Here's how the part is built. I have some questions about the finished solid (model axes, mm). A direction names the side the tool comes from. Round coordinates to 2 decimals unless told otherwise and drop trailing zeros. Order: outer loops, then holes, each group sorted by start corner. A loop starts at its lowest first (then second) coordinate and runs counter-clockwise, first axis right, second up. Notation, with made-up numbers: (72.25, 31) -> (121.25, 31) arc R24 ccw to (121.25, 57) -> close; hole circle Ø8 at (-38, 58). An arc over 180 degrees is marked (long way). Answer in a Markdown table with one row per item.
```python
from build123d import *

# Parameters (mm, degrees)
SKETCH2_W           = 16
SKETCH2_H           = 16
BOSS_EXTRUDE1_DEPTH = 1.7
SKETCH3_R           = 0.75
CUT_EXTRUDE1_DEPTH  = 1.7
SKETCH4_W           = 3
SKETCH4_H           = 3
BOSS_EXTRUDE2_DEPTH = 1
SKETCH5_W           = 0.710598353
SKETCH5_H           = 2.069095202
SKETCH5_H_2         = 1.860095687
BOSS_EXTRUDE3_DEPTH = 0.5
SKETCH6_R           = 1.65
CUT_EXTRUDE2_DEPTH  = 12.440716761


with BuildPart() as part:
    # Sketch2 → Boss-Extrude1 (new body)
    with BuildSketch(Plane(origin=(0, 0, 0), x_dir=(1, 0, 0), z_dir=(0, 1, 0))):
        Rectangle(SKETCH2_W, SKETCH2_H)
    extrude(amount=BOSS_EXTRUDE1_DEPTH)

    # Sketch3 → Cut-Extrude1 (cut)
    with BuildSketch(Plane(origin=(0, 1.7, 0), x_dir=(1, 0, 0), z_dir=(0, 1, 0))):
        with Locations(Location((-6.5, 6.35, 0), (0, 0, 270))):
            Circle(SKETCH3_R)
        with Locations(Location((-6.5, 3.81, 0), (0, 0, 270))):
            Circle(SKETCH3_R)
        with Locations(Location((-6.5, 1.27, 0), (0, 0, 270))):
            Circle(SKETCH3_R)
        with Locations(Location((-6.5, -1.27, 0), (0, 0, 270))):
            Circle(SKETCH3_R)
        with Locations(Location((-6.5, -3.81, 0), (0, 0, 270))):
            Circle(SKETCH3_R)
        with Locations(Location((-6.5, -6.35, 0), (0, 0, 270))):
            Circle(SKETCH3_R)
    extrude(amount=-CUT_EXTRUDE1_DEPTH, mode=Mode.SUBTRACT)

    # Sketch4 → Boss-Extrude2 (add)
    with BuildSketch(Plane(origin=(0, 1.7, 0), x_dir=(1, 0, 0), z_dir=(0, 1, 0))):
        Rectangle(SKETCH4_W, SKETCH4_H)
    extrude(amount=BOSS_EXTRUDE2_DEPTH)

    # Sketch5 → Boss-Extrude3 (add)
    with BuildSketch(Plane(origin=(0, 1.7, 0), x_dir=(1, 0, 0), z_dir=(0, 1, 0))):
        with Locations((0.571550994, 4.723389047)):
            Rectangle(SKETCH5_W, SKETCH5_H)
        with Locations((-0.428449007, 4.723389047)):
            Rectangle(SKETCH5_W, SKETCH5_H)
        with Locations((-1.01364765, -4.388989823)):
            Rectangle(SKETCH5_W, SKETCH5_H_2)
        with Locations((-0.013647649, -4.388989823)):
            Rectangle(SKETCH5_W, SKETCH5_H_2)
        with Locations((0.986352351, -4.388989823)):
            Rectangle(SKETCH5_W, SKETCH5_H_2)
    extrude(amount=BOSS_EXTRUDE3_DEPTH)

    # Sketch6 → Cut-Extrude2 (cut, through all)
    with BuildSketch(Plane(origin=(0, 1.7, 0), x_dir=(1, 0, 0), z_dir=(0, 1, 0))):
        with Locations(Location((5, 5.1, 0), (0, 0, 270))):
            Circle(SKETCH6_R)
        with Locations(Location((5, -5.1, 0), (0, 0, 90))):
            Circle(SKETCH6_R)
    extrude(amount=-CUT_EXTRUDE2_DEPTH, mode=Mode.SUBTRACT)


solid = part.part
```
1. Suppose I cut it at D-D on y = 1.2. State how many separate pieces and enclosed holes the cut face has, then the cut area to 3 significant figures.
Numbers:
| item | result |
|---|---|
| separate pieces | 1 |
| enclosed holes | 8 |
| area | 228 mm2 |
2. For faces 5 (the face through (-6.47, 0.86, 3.06)), 6 (the face through (0, 2, -1.5)), 7 (the face through (1.5, 2, 0)), 8 (the face through (-1.5, 2, 0)), which set-ups out of +Z, -Z, +X, -X, +Y, -Y let a thin tool reach every point of the face, with its end or its side?
Numbers:
| item | result |
|---|---|
| face 5 | +Y, -Y |
| face 6 | +X, -X, +Y |
| face 7 | +Z, -Z, +X, +Y |
| face 8 | +Z, -Z, -X, +Y |
3. Suppose I cut it at A-A on z = 1.27. Write out the boundary of the cut face in (x, y).
Numbers:
| item | result |
|---|---|
| outline | (-8, 0) -> (-7.25, 0) -> (-7.25, 1.7) -> (-8, 1.7) -> close; (-5.75, 0) -> (8, 0) -> (8, 1.7) -> (1.5, 1.7) -> (1.5, 2.7) -> (-1.5, 2.7) -> (-1.5, 1.7) -> (-5.75, 1.7) -> close |
4. Suppose I cut it at C-C on x = -6.5. Write out the boundary of the cut face in (y, z), then the cut area to 3 significant figures.
Numbers:
| item | result |
|---|---|
| outline | (0, -8) -> (1.7, -8) -> (1.7, -7.1) -> (0, -7.1) -> close; (0, -5.6) -> (1.7, -5.6) -> (1.7, -4.56) -> (0, -4.56) -> close; (0, -3.06) -> (1.7, -3.06) -> (1.7, -2.02) -> (0, -2.02) -> close; (0, -0.52) -> (1.7, -0.52) -> (1.7, 0.52) -> (0, 0.52) -> close; (0, 2.02) -> (1.7, 2.02) -> (1.7, 3.06) -> (0, 3.06) -> close; (0, 4.56) -> (1.7, 4.56) -> (1.7, 5.6) -> (0, 5.6) -> close; (0, 7.1) -> (1.7, 7.1) -> (1.7, 8) -> (0, 8) -> close |
| area | 11.9 mm2 |
5. For pin 1 Ø4 at (x, z) = (1, -5.5) entering from +Y; pin 2 Ø0.5 at (x, y) = (0.5, 2) entering from +Z, each with a flat end and sliding along its axis, tell me the tip position at first contact or that it passes through.
Numbers:
| item | result |
|---|---|
| pin 1 | stops at y = 2.2 |
| pin 2 | stops at z = 5.32 |
6. Please list where these lines run through material, in increasing order: line 1 along X through (y, z) = (0.55, -5.1); line 2 along X through (y, z) = (0.7, -3.81); line 3 along Z through (x, y) = (-1, 2.1).
Numbers:
| item | result |
|---|---|
| line 1 | x = -8 to 3.35, 6.65 to 8 |
| line 2 | x = -8 to -7.25, -5.75 to 3.97, 6.03 to 8 |
| line 3 | z = -1.5 to 1.5, 3.46 to 5.32 |
7. We'd pull the mould along Z, two halves only. Please class faces 1 (the face through (0, 2.7, 0)), 2 (the face through (5.632, 0.862, 3.576)), 3 (the face through (0, 1, -8)), 4 (the face through (-6.79, 0.86, 7.04)): released by +Z, released by -Z, zero draft, split by the parting line, or undercut.
Numbers:
| item | result |
|---|---|
| face 1 | zero draft |
| face 2 | undercut |
| face 3 | released by -Z |
| face 4 | undercut |
8. Suppose I cut it at B-B on y = 2. Write out the boundary of the cut face in (x, z), then the cut area to 3 significant figures.
Numbers:
| item | result |
|---|---|
| outline | (-1.5, -1.5) -> (1.5, -1.5) -> (1.5, 1.5) -> (-1.5, 1.5) -> close; (-1.37, 3.46) -> (-0.66, 3.46) -> (-0.66, 5.32) -> (-1.37, 5.32) -> close; (-0.78, -5.76) -> (-0.07, -5.76) -> (-0.07, -3.69) -> (-0.78, -3.69) -> close; (-0.37, 3.46) -> (0.34, 3.46) -> (0.34, 5.32) -> (-0.37, 5.32) -> close; (0.22, -5.76) -> (0.93, -5.76) -> (0.93, -3.69) -> (0.22, -3.69) -> close; (0.63, 3.46) -> (1.34, 3.46) -> (1.34, 5.32) -> (0.63, 5.32) -> close |
| area | 15.9 mm2 |
